```python
from build123d import *

# Parameters (mm, degrees)
BOSS_EXTRUDE1_DEPTH = 25.4
SKETCH3_R           = 1.7272
CUT_EXTRUDE2_DEPTH  = 26.4


with BuildPart() as part:
    # Sketch1 → Boss-Extrude1 (new body)
    with BuildSketch(Plane(origin=(0, 0, 0), x_dir=(1, 0, 0), z_dir=(0, 1, 0))):
        Polygon((-2.767735883, 3.334911674), (-1.744793251, 6.855482892), (-4.282226046, 9.501662807), (-7.842601473, 8.627271504), (-8.865544105, 5.106700285), (-6.32811131, 2.46052037), align=None)
    extrude(amount=BOSS_EXTRUDE1_DEPTH)

    # Sketch3 → Cut-Extrude2 (cut, through all)
    with BuildSketch(Plane.XZ):
        with Locations((-5.305168678, -5.981091589)):
            Circle(SKETCH3_R)
    extrude(amount=-CUT_EXTRUDE2_DEPTH, mode=Mode.SUBTRACT)


solid = part.part
```
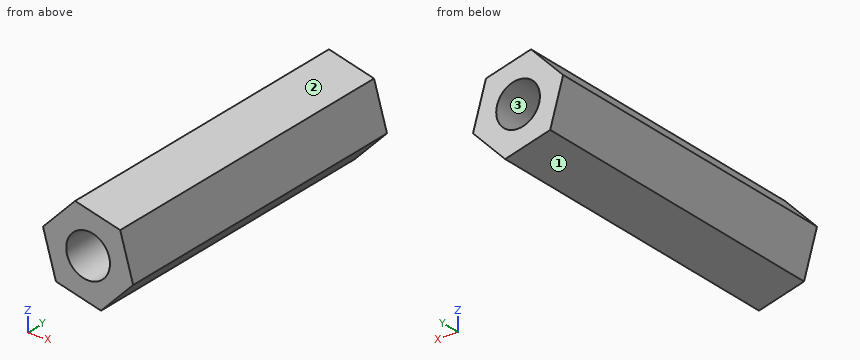
The listing builds one solid part. Answer for the finished solid, in the listing's coordinates (mm). Face numbers are marked on the shaded views. Round coordinates to 2 decimals unless told otherwise and drop trailing zeros. Write each loop counter-clockwise with the first axis right and the second up, starting at its lowest first coordinate (ties: lowest second). Pieces come first, ordered by that corner, then holes. Notation, with made-up numbers: (-29, -7.75) -> (3, -7.75) arc R18 ccw to (3, 23.25) -> close; hole circle Ø2 at (55.25, 86.25). An arc over 180 degrees is marked (long way). Answer as a JSON object with one key per item and string values. Group by question number.
Q1. Section D-D (z = -2.75) is taken. Write down the section's boundary in (x, y).
Q2. Section A-A (x = -4) is taken. Write down the section's boundary in (y, z), plus the area to 3 significant figures.
Q3. Section B-B (y = 10.25) is taken. Write down the section's boundary in (x, z), plus the area to 3 significant figures.
Q4. Section C-C (z = -6.5) is taken. Write down the section's boundary in (x, y).
Q5. Each of these flat-tipped pins is pushed along its axis until it touches: pin 1 Ø1 at (y, z) = (17, -4.5) entering from +X; pin 2 Ø1 at (y, z) = (21, -3.5) entering from +X. Where does it stop, or does it pass through?
Q6. Straight lines are drawn through the part: line 1 along X through (y, z) = (15.5, -6.25); line 2 along Z through (x, y) = (-5.5, 5.5); line 3 along X through (y, z) = (16, -8.25). For each, find the intervals that lie inside material, in ascending order.
Q7. Determine the mould class of the marked faces 1, 2 and 3 for opening direction Z: pulls with the +Z half, pulls with the -Z half, needs draft (parallel to the pull), parting line crosses it, or undercut.
Check values:
{
 "1": {"outline": "(-6.61, 0) -> (-5.15, 0) -> (-5.15, 25.4) -> (-6.61, 25.4) -> close"},
 "2": {"outline": "(0, -9.21) -> (25.4, -9.21) -> (25.4, -7.11) -> (0, -7.11) -> close; (0, -4.85) -> (25.4, -4.85) -> (25.4, -3.03) -> (0, -3.03) -> close", "area": "99.4 mm^2"},
 "3": {"outline": "(-8.87, -5.11) -> (-7.84, -8.63) -> (-4.28, -9.5) -> (-1.74, -6.86) -> (-2.77, -3.33) -> (-6.33, -2.46) -> close; hole circle Ø3.45 at (-5.31, -5.98)", "area": "25.5 mm^2"},
 "4": {"outline": "(-8.46, 0) -> (-6.95, 0) -> (-6.95, 25.4) -> (-8.46, 25.4) -> close; (-3.66, 0) -> (-1.85, 0) -> (-1.85, 25.4) -> (-3.66, 25.4) -> close"},
 "5": {"pin 1": "x = -2.28", "pin 2": "x = -2.57"},
 "6": {"line 1": "-8.53 to -7.01, -3.6 to -1.92", "line 2": "-9.2 to -7.7, -4.26 to -2.66", "line 3": "-7.95 to -3.08"},
 "7": {"face 1": "pulls with the -Z half", "face 2": "pulls with the +Z half", "face 3": "undercut"}
}
